```python
from build123d import *

# Parameters (mm, degrees)
SKIZZE1_W                       = 200
SKIZZE1_H                       = 200
AUFSATZ_LINEAR_AUSTRAGEN1_DEPTH = 20
SKIZZE2_R                       = 50
SKIZZE2_R_2                     = 37.5
AUFSATZ_LINEAR_AUSTRAGEN2_DEPTH = 50
FASE1_SIZE                      = 50
SKIZZE3_R                       = 7.5
SCHNITT_LINEAR_AUSTRAGEN1_DEPTH = 50


with BuildPart() as part:
    # Skizze1 → Aufsatz-Linear austragen1 (new body)
    with BuildSketch(Plane(origin=(0, 0, 0), x_dir=(1, 0, 0), z_dir=(0, 1, 0))):
        Rectangle(SKIZZE1_W, SKIZZE1_H)
    extrude(amount=AUFSATZ_LINEAR_AUSTRAGEN1_DEPTH)

    # Skizze2 → Aufsatz-Linear austragen2 (add)
    with BuildSketch(Plane(origin=(0, 20, 0), x_dir=(1, 0, 0), z_dir=(0, 1, 0))):
        with Locations(Location((0, 0, 0), (0, 0, 90))):
            Circle(SKIZZE2_R)
        with Locations(Location((0, 0, 0), (0, 0, 270))):
            Circle(SKIZZE2_R_2, mode=Mode.SUBTRACT)
    extrude(amount=AUFSATZ_LINEAR_AUSTRAGEN2_DEPTH)

    # Fase1
    fase1_edges = [part.edges().sort_by_distance(p)[0] for p in [
        (0, 20, 50),
    ]]
    chamfer(fase1_edges, length=FASE1_SIZE - 0.0001)  # a hair under: the kernel refuses the full size

    # Skizze3 → Schnitt-Linear austragen1 (cut)
    with BuildSketch(Plane(origin=(0, 20, 0), x_dir=(1, 0, 0), z_dir=(0, 1, 0))):
        with Locations(Location((85, 85, 0), (0, 0, 270))):
            Circle(SKIZZE3_R)
        with Locations(Location((-85, 85, 0), (0, 0, 90))):
            Circle(SKIZZE3_R)
        with Locations(Location((85, -85, 0), (0, 0, 90))):
            Circle(SKIZZE3_R)
        with Locations(Location((-85, -85, 0), (0, 0, 270))):
            Circle(SKIZZE3_R)
    extrude(amount=-SCHNITT_LINEAR_AUSTRAGEN1_DEPTH, mode=Mode.SUBTRACT)


solid = part.part
```
Could you check a few things on this model? Use its own coordinates, in mm. A direction names the side the tool comes from. Coordinates: 2 decimals unless noted, no trailing zeros. Write each loop counter-clockwise with the first axis right and the second up, starting at its lowest first coordinate (ties: lowest second). Pieces come first, ordered by that corner, then holes. Notation, with made-up numbers: (63.25, 34) -> (75.25, 34) arc R21 cw to (75.25, 39) -> close; hole circle Ø4 at (62.25, 71.25). An arc over 180 degrees is marked (long way). One line per question, with ' | ' between items. Start each with the question number.
1. For faces 1 (the face through (-60, 20, 81)), 2 (the face through (-92.32, 10.14, 83.37)), which set-ups out of +Z, -Z, +X, -X, +Y, -Y let a thin tool reach every point of the face, with its end or its side?
2. If we section it at D-D (x = 85): Count the separate pieces of the cut face and the enclosed holes in it, and give its area (3 significant figures).
3. Will these pins go through, and if not, where does the flat tip stop? P1, Ø12, axis at x = 85, z = -85, coming from the +Y side; P2, Ø1, axis at y = 44, z = 26.5, coming from the +X side; P3, Ø19.5, axis at x = -85, z = -85, coming from the +Y side; P4, Ø1.5, axis at y = 41, z = -11, coming from the -X side.
4. If we section it at A-A (y = 15): Please give me the cut outline in (x, z).
5. Please list where these lines run through material, in increasing order: line 1 along X through (y, z) = (16, -85); line 2 along X through (y, z) = (43, -4.5); line 3 along Y through (x, z) = (8, -16.5).
6. Thinking about a two-plate mould opening in X: for faces 3 (the face through (91.654, 10.14, 81.539)), 4 (the face through (-1, 0, -1)), 5 (the face through (31.901, 67.572, 41.605)), which applies, pulls with the +X half, pulls with the -X half, needs draft (parallel to the pull), parting line crosses it, or undercut?
Return value:
1) face 1: +Y | face 2: +Y, -Y
2) separate pieces: 3 | enclosed holes: 0 | area: 4,440 mm²
3) P1: passes through | P2: stops at x = 71.79 | P3: stops at y = 20 | P4: stops at x = -78.99
4) outline: (-100, -100) -> (100, -100) -> (100, 100) -> (-100, 100) -> close; hole circle Ø15 at (-85, -85); hole circle Ø15 at (-85, 85); hole circle Ø15 at (85, -85); hole circle Ø15 at (85, 85)
5) line 1: x = -100 to -92.5, -77.5 to 77.5, 92.5 to 100 | line 2: x = -76.87 to -37.23, 37.23 to 76.87 | line 3: y = 0 to 20
6) face 3: undercut | face 4: needs draft | face 5: parting line crosses it
